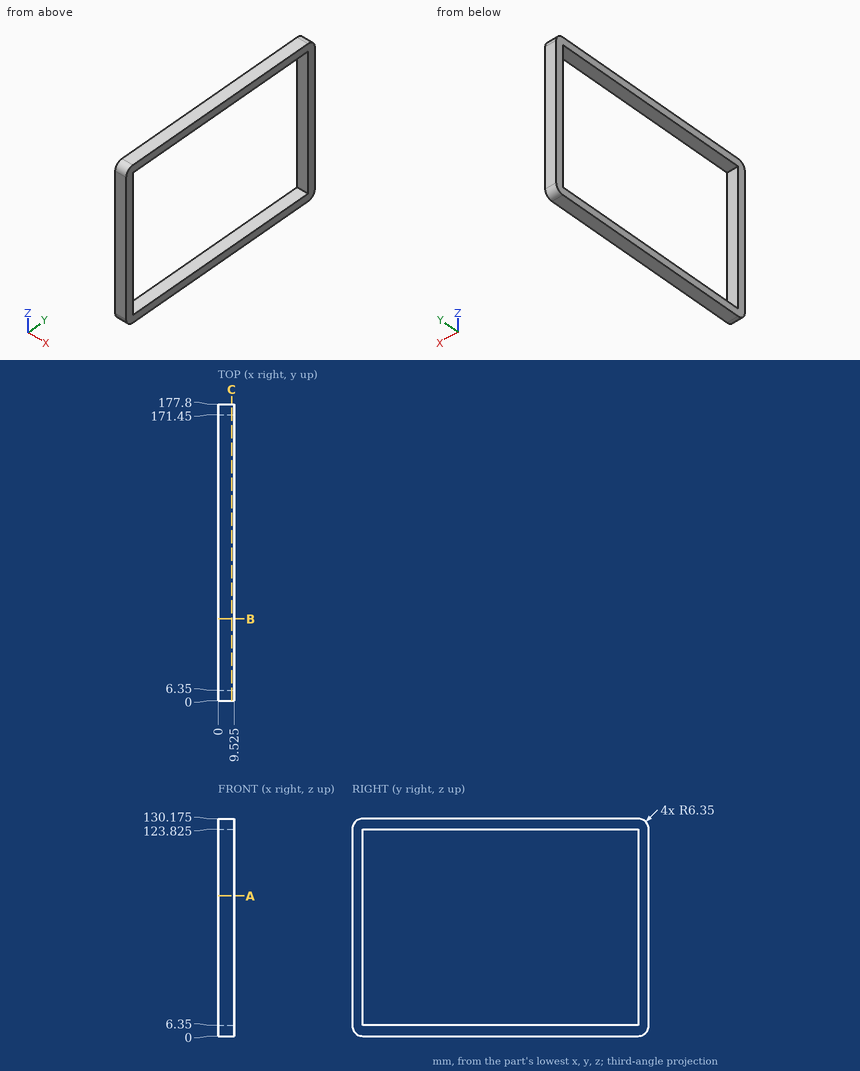
Answer from the drawing. Dimensions are ordinates in mm from the lowest x, y and z of the part. Coordinates: 2 decimals unless noted, no trailing zeros. Write each loop counter-clockwise with the first axis right and the second up, starting at its lowest first coordinate (ties: lowest second). Pieces come first, ordered by that corner, then holes. Notation, with made-up numbers: M 19,29.5 L 29,29.5 A26 cw 29,45.5 Z; hole C 53,44.5 d1. An arc over 180 degrees is marked long. Use one line per item in the form item = value. Start each with the question number.
1. Straight lines are drawn through the part: probe 1 along Y at (x, z) = (2.5, 106); probe 2 along Z at (x, y) = (7, 144.5) (3 decimals). For each, find the intervals that lie inside material, in ascending order. Write a range as from..to.
2. The part is cut by section B-B (y = 49). Give the vertices of the cut face in (x, z) (3 decimals), plus the area to 3 significant figures.
3. The part is cut by section A-A (z = 84). Give the vertices of the cut face in (x, y) (3 decimals), plus the area to 3 significant figures.
4. The part is cut by section C-C (x = 8). Give the vertices of the cut face in (y, z) (3 decimals), plus the area to 3 significant figures.
Evaluation:
q1.probe_1 = 0..6.35, 171.45..177.8
q1.probe_2 = 0..6.35, 123.825..130.175
q2.outline = M 0,0 L 9.525,0 L 9.525,6.35 L 0,6.35 Z; M 0,123.825 L 9.525,123.825 L 9.525,130.175 L 0,130.175 Z
q2.area = 121 mm^2
q3.outline = M 0,0 L 9.525,0 L 9.525,6.35 L 0,6.35 Z; M 0,171.45 L 9.525,171.45 L 9.525,177.8 L 0,177.8 Z
q3.area = 121 mm^2
q4.outline = M 0,6.35 A6.35 ccw 6.35,0 L 171.45,0 A6.35 ccw 177.8,6.35 L 177.8,123.825 A6.35 ccw 171.45,130.175 L 6.35,130.175 A6.35 ccw 0,123.825 Z; hole M 6.35,6.35 L 171.45,6.35 L 171.45,123.825 L 6.35,123.825 Z
q4.area = 3,720 mm^2
